For this review, take the finished solid that the model builds, in its own axes (mm). Round coordinates to 2 decimals unless told otherwise and drop trailing zeros. Write each loop counter-clockwise with the first axis right and the second up, starting at its lowest first coordinate (ties: lowest second). Pieces come first, ordered by that corner, then holes. Notation, with made-up numbers: (31.5, 36.5) -> (67.5, 36.5) arc R31 cw to (67.5, 71.5) -> close; hole circle Ø8 at (-29.75, -21.5). An arc over 180 degrees is marked (long way). Answer in a Markdown table with one row per item.
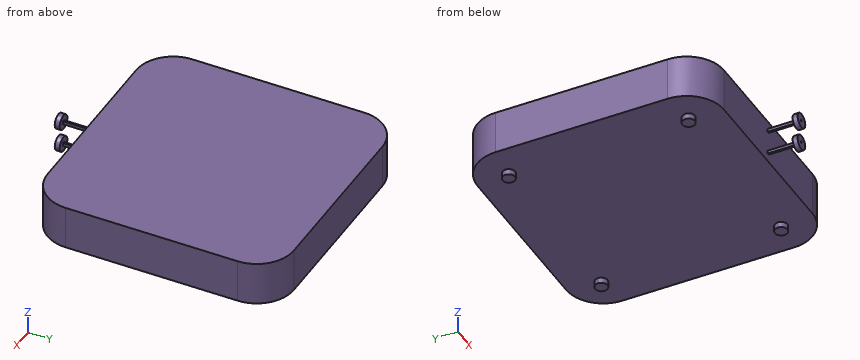
from build123d import *

# Parameters (mm, degrees)
F1_DEPTH = 28.1
F2_DEPTH = 35.5
F4_DEPTH = 42.5
F5_R     = 9.525
F6_DEPTH = 6.35
F7_R     = 9.525
F8_DEPTH = 6.35


with BuildPart() as f1:
    # F0 (on Top) → F1 (new body, symmetric)
    with BuildSketch(Plane.XY):
        with BuildLine():
            Line((107, -115), (0, -115))
            Line((0, -115), (0, -157.5))
            Line((0, -157.5), (110, -157.5))
            ThreePointArc((110, -157.5), (143.5875721064, -143.5875721064), (157.5, -110))
            Line((157.5, -110), (157.5, 0))
            Line((157.5, 0), (115, 0))
            Line((115, 0), (115, -107))
            ThreePointArc((115, -107), (120.6568542495, -109.3431457505), (123, -115))
            ThreePointArc((123, -115), (115, -123), (107, -115))
        make_face()
        with BuildLine():
            Line((115, 0), (0, 0))
            Line((0, 0), (0, -115))
            Line((0, -115), (107, -115))
            ThreePointArc((107, -115), (109.3431457505, -109.3431457505), (115, -107))
            Line((115, -107), (115, 0))
        make_face()
        with BuildLine():
            Line((115, 107), (115, 0))
            Line((115, 0), (157.5, 0))
            Line((157.5, 0), (157.5, 110))
            ThreePointArc((157.5, 110), (143.5875721064, 143.5875721064), (110, 157.5))
            Line((110, 157.5), (0, 157.5))
            Line((0, 157.5), (0, 142.7501142025))
            Line((0, 142.7501142025), (0, 115))
            Line((0, 115), (107, 115))
            ThreePointArc((107, 115), (115, 123), (123, 115))
            ThreePointArc((123, 115), (120.6568542495, 109.3431457505), (115, 107))
        make_face()
        with BuildLine():
            Line((0, 115), (0, 0))
            Line((0, 0), (115, 0))
            Line((115, 0), (115, 107))
            ThreePointArc((115, 107), (109.3431457505, 109.3431457505), (107, 115))
            Line((107, 115), (0, 115))
        make_face()
        with BuildLine():
            Line((-115, 0), (0, 0))
            Line((0, 0), (0, 115))
            Line((0, 115), (-107, 115))
            ThreePointArc((-107, 115), (-109.3431457505, 109.3431457505), (-115, 107))
            Line((-115, 107), (-115, 0))
        make_face()
        with BuildLine():
            Line((-157.5, 0), (-115, 0))
            Line((-115, 0), (-115, 107))
            ThreePointArc((-115, 107), (-120.6568542495, 120.6568542495), (-107, 115))
            Line((-107, 115), (0, 115))
            Line((0, 115), (0, 142.7501142025))
            Line((0, 142.7501142025), (0, 157.5))
            Line((0, 157.5), (-110, 157.5))
            ThreePointArc((-110, 157.5), (-143.5875721064, 143.5875721064), (-157.5, 110))
            Line((-157.5, 110), (-157.5, 0))
        make_face()
        with BuildLine():
            Line((0, -115), (0, 0))
            Line((0, 0), (-115, 0))
            Line((-115, 0), (-115, -107))
            ThreePointArc((-115, -107), (-109.3431457505, -109.3431457505), (-107, -115))
            Line((-107, -115), (0, -115))
        make_face()
        with BuildLine():
            Line((0, -157.5), (0, -115))
            Line((0, -115), (-107, -115))
            ThreePointArc((-107, -115), (-120.6568542495, -120.6568542495), (-115, -107))
            Line((-115, -107), (-115, 0))
            Line((-115, 0), (-157.5, 0))
            Line((-157.5, 0), (-157.5, -110))
            ThreePointArc((-157.5, -110), (-143.5875721064, -143.5875721064), (-110, -157.5))
            Line((-110, -157.5), (0, -157.5))
        make_face()
        with BuildLine():
            Line((115, -115), (107, -115))
            ThreePointArc((107, -115), (115, -123), (123, -115))
            ThreePointArc((123, -115), (120.6568542495, -109.3431457505), (115, -107))
            Line((115, -107), (115, -115))
        make_face()
        with BuildLine():
            ThreePointArc((115, -107), (109.3431457505, -109.3431457505), (107, -115))
            Line((107, -115), (115, -115))
            Line((115, -115), (115, -107))
        make_face()
        with BuildLine():
            ThreePointArc((-115, -107), (-120.6568542495, -120.6568542495), (-107, -115))
            Line((-107, -115), (-115, -115))
            Line((-115, -115), (-115, -107))
        make_face()
        with BuildLine():
            Line((-115, -115), (-107, -115))
            ThreePointArc((-107, -115), (-109.3431457505, -109.3431457505), (-115, -107))
            Line((-115, -107), (-115, -115))
        make_face()
        with BuildLine():
            Line((115, 115), (115, 107))
            ThreePointArc((115, 107), (120.6568542495, 109.3431457505), (123, 115))
            ThreePointArc((123, 115), (115, 123), (107, 115))
            Line((107, 115), (115, 115))
        make_face()
        with BuildLine():
            ThreePointArc((107, 115), (109.3431457505, 109.3431457505), (115, 107))
            Line((115, 107), (115, 115))
            Line((115, 115), (107, 115))
        make_face()
        with BuildLine():
            ThreePointArc((-107, 115), (-120.6568542495, 120.6568542495), (-115, 107))
            Line((-115, 107), (-115, 115))
            Line((-115, 115), (-107, 115))
        make_face()
        with BuildLine():
            Line((-115, 115), (-115, 107))
            ThreePointArc((-115, 107), (-109.3431457505, 109.3431457505), (-107, 115))
            Line((-107, 115), (-115, 115))
        make_face()
    extrude(amount=F1_DEPTH, both=True)

    # F0 (on Top) → F2 (join)
    with BuildSketch(Plane.XY):
        with BuildLine():
            ThreePointArc((-115, -107), (-120.6568542495, -120.6568542495), (-107, -115))
            Line((-107, -115), (-115, -115))
            Line((-115, -115), (-115, -107))
        make_face()
        with BuildLine():
            Line((-115, -115), (-107, -115))
            ThreePointArc((-107, -115), (-109.3431457505, -109.3431457505), (-115, -107))
            Line((-115, -107), (-115, -115))
        make_face()
        with BuildLine():
            Line((115, -115), (107, -115))
            ThreePointArc((107, -115), (115, -123), (123, -115))
            ThreePointArc((123, -115), (120.6568542495, -109.3431457505), (115, -107))
            Line((115, -107), (115, -115))
        make_face()
        with BuildLine():
            ThreePointArc((115, -107), (109.3431457505, -109.3431457505), (107, -115))
            Line((107, -115), (115, -115))
            Line((115, -115), (115, -107))
        make_face()
        with BuildLine():
            Line((115, 115), (115, 107))
            ThreePointArc((115, 107), (120.6568542495, 109.3431457505), (123, 115))
            ThreePointArc((123, 115), (115, 123), (107, 115))
            Line((107, 115), (115, 115))
        make_face()
        with BuildLine():
            ThreePointArc((107, 115), (109.3431457505, 109.3431457505), (115, 107))
            Line((115, 107), (115, 115))
            Line((115, 115), (107, 115))
        make_face()
        with BuildLine():
            ThreePointArc((-107, 115), (-120.6568542495, 120.6568542495), (-115, 107))
            Line((-115, 107), (-115, 115))
            Line((-115, 115), (-107, 115))
        make_face()
        with BuildLine():
            Line((-115, 115), (-115, 107))
            ThreePointArc((-115, 107), (-109.3431457505, 109.3431457505), (-107, 115))
            Line((-107, 115), (-115, 115))
        make_face()
    extrude(amount=-F2_DEPTH)

    # F3 (on face) → F4 (join)
    with BuildSketch(Plane.XZ.offset(157.5)):
        Polygon((0, -13.95), (0, -13.45), (-1.275, -13.45), (-1.275, -17.55), (1.275, -17.55), (1.275, -15.5), (0.775, -15.5), (0.775, -17.05), (-0.775, -17.05), (-0.775, -13.95), align=None)
        Polygon((1.275, -13.45), (0, -13.45), (0, -13.95), (0.775, -13.95), (0.775, -15.5), (1.275, -15.5), align=None)
        Polygon((-1.275, 13.45), (0, 13.45), (0, 13.95), (-0.775, 13.95), (-0.775, 17.05), (0.775, 17.05), (0.775, 15.5), (1.275, 15.5), (1.275, 17.55), (-1.275, 17.55), align=None)
        Polygon((0, 13.95), (0, 13.45), (1.275, 13.45), (1.275, 15.5), (0.775, 15.5), (0.775, 13.95), align=None)
    extrude(amount=F4_DEPTH)

    # F5 (on face) → F6 (join)
    with BuildSketch(Plane.XZ.offset(200)):
        with Locations((0, 15.5)):
            Circle(F5_R)
        Polygon((-1.275, 13.45), (-1.275, 15.5), (-1.275, 17.55), (0, 17.55), (1.275, 17.55), (1.275, 15.5), (1.275, 13.45), (0, 13.45), align=None, mode=Mode.SUBTRACT)
    extrude(amount=-F6_DEPTH)

    # F7 (on face) → F8 (join)
    with BuildSketch(Plane.XZ.offset(200)):
        with Locations((0, -15.5)):
            Circle(F7_R)
        Polygon((-1.275, -17.55), (-1.275, -15.5), (-1.275, -13.45), (0, -13.45), (1.275, -13.45), (1.275, -15.5), (1.275, -17.55), (0, -17.55), align=None, mode=Mode.SUBTRACT)
    extrude(amount=-F8_DEPTH)


solid = f1.part
1) Consider section A-A on y = 100.5. State the section outline as (x, z) points, then the cut area to 3 significant figures.
Solved:
| item | result |
|---|---|
| outline | (-157.5, -28.1) -> (157.5, -28.1) -> (157.5, 28.1) -> (-157.5, 28.1) -> close |
| area | 17,700 mm² |
2) Clearance check with flat-ended pins moving along their axes: pin 1 Ø2 at (x, y) = (0.5, -173) entering from +Z; pin 2 Ø3.5 at (y, z) = (-183, 15.5) entering from +X (3 decimals); pin 3 Ø2 at (y, z) = (-171, -15) entering from -X (3 decimals). State where each tip first meets the part, or that it passes through.
Solved:
| item | result |
|---|---|
| pin 1 | z = 17.55 |
| pin 2 | x = 1.275 |
| pin 3 | x = -1.275 |
3) For line 1 (Z direction, x = 106, y = 50.5); line 2 (Y direction, x = 19.5, z = 24.5); line 3 (Y direction, x = 1, z = 12), list the stretches that pass through material, from the lowest coordinate up. Write a range as [from, to].
Solved:
| item | result |
|---|---|
| line 1 | [-28.1, 28.1] |
| line 2 | [-157.5, 157.5] |
| line 3 | [-200, -193.65], [-157.5, 157.5] |
